Autodesk Inventor part; units mm, degrees
ref_plane "YZ Plane" through (0, 0, 0) normal (1, 0, 0) x (0, 1, 0)
ref_plane "XZ Plane" through (0, 0, 0) normal (0, 1, 0) x (-1, 0, 0)
ref_plane "XY Plane" through (0, 0, 0) normal (0, 0, 1) x (1, 0, 0)
sketch "Sketch1" plane through (0, 0, 0) normal (0, 1, 0) x (-1, 0, 0)
  circle A0 centre (0, 0) radius 25
  circle A1 centre (-200, 0) radius 25
  line L0 (0, 25) -> (-200, 25)
  line L1 (-200, 25) -> (-200, -25)
  line L2 (-200, -25) -> (0, -25)
  line L3 (0, -25) -> (0, 25)
  point P0 (-200, 0)
  point P1 (0, 0)
  point P2 (0, -25)
  dimension "d0" = 50
  dimension "d1" = 50
  dimension "d2" = 200
extrude "Extrusion1" add sketch "Sketch1" along normal mid plane 20
sketch "Sketch4" plane through (0, 0, 0) normal (0, 1, 0) x (-1, 0, 0)
  arc A0 (0, -25) -> (0, 25) centre (0, 0) ccw
  line L0 (0, -25) -> (-200, -25)
  arc A1 (-200, 25) -> (-200, -25) centre (-200, 0) ccw
  line L1 (-200, 25) -> (0, 25)
  line L2 (0, -25) -> (-200, -25)
  line L3 (-80, -25) -> (-80, 25)
  line L4 (-200, 25) -> (0, 25)
  dimension "d10" = 80
extrude "Extrusion3" add sketch "Sketch4" along normal mid plane 50 contours L0 L3 L1 A0
sketch "Sketch6" plane through (0, 0, 0) normal (0, 1, 0) x (-1, 0, 0)
  circle A0 centre (0, 0) radius 15
  arc A1 (-200, 25) -> (-200, -25) centre (-200, 0) ccw
  circle A2 centre (-200, 0) radius 15
  line L0 (0, -25) -> (-80, -25)
  line L1 (-65, -25) -> (-65, 25)
  arc A3 (0, -25) -> (0, 25) centre (0, 0) ccw
  line L2 (-80, 25) -> (0, 25)
  point P0 (-65, 0)
  point P1 (25, 0)
  dimension "d13" = 30
  dimension "d14" = 30
  dimension "d16" = 90
extrude "Extrusion4" cut sketch "Sketch6" along normal mid plane 20
properties part number "Manipulator Link"
Could you check a few things on this model? Use its own coordinates, in mm. A direction names the side the tool comes from. Give positions to 0.01 mm unless a question says otherwise; leave off trailing zeros. Loops run counter-clockwise (first coordinate to the right, second up) from the corner with the lowest first, then second, coordinate; pieces in that order, holes last. Notation, with made-up numbers: M 55,76 L 88,76 A23 cw 88,92 Z; hole C 67.5,-3 d11. An arc over 180 degrees is marked long. Answer as a JSON object with one key per item and string values.
Q1. If I drill on probe 1 along X at (y, z) = (3, 1); probe 2 along Z at (x, y) = (200, 1); probe 3 along Y at (x, z) = (9.5, -12.5), over which ranges is the centre line in solid material (lowest first)? Write a range as [from, to].
Values found:
{"probe 1": "x = [-14.97, 14.97], [65, 185.03], [214.97, 224.98]", "probe 2": "z = [-25, -15], [15, 25]", "probe 3": "y = [-25, -10], [10, 25]"}
Q2. Suppose I cut it at D-D, the plane x = 165.5. List the corners of the cut face in (y, z) for me.
Values found:
{"outline": "M -10,-25 L 10,-25 L 10,25 L -10,25 Z"}
Q3. For P1, Ø3, axis at y = -12.5, z = 0.5, coming from the +X side; P2, Ø8, axis at x = 150, z = 2, coming from the +Y side; P3, Ø6, axis at y = 1.5, z = 12, coming from the -X side, each with a flat end and sliding along its axis, tell me the tip position at first contact or that it passes through.
Values found:
{"P1": "stops at x = 80", "P2": "stops at y = 10", "P3": "stops at x = -12"}
Q4. If we mould it in two halves opening along Y, with no side actions, what happens to faces 1 (the cylindrical face through (224.994, -0.14, -0.55)), 2 (the flat face through (154, 10, 0)), 3 (the flat face through (31, 10, 0))? For each: pulls with the +Y half, pulls with the -Y half, needs draft (parallel to the pull), parting line crosses it, or undercut.
Values found:
{"face 1": "needs draft", "face 2": "pulls with the +Y half", "face 3": "undercut"}
Q5. Suppose I cut it at A-A, the plane z = 0. List the corners of the cut face in (x, y) for me.
Values found:
{"outline": "M -25,-25 L 80,-25 L 80,-10 L 185,-10 L 185,10 L 80,10 L 80,25 L -25,25 L -25,10 L -15,10 L -15,-10 L -25,-10 Z; M 215,-10 L 225,-10 L 225,10 L 215,10 Z; hole M 15,-10 L 65,-10 L 65,10 L 15,10 Z"}
Q6. For faces 4 (the cylindrical face through (14.985, -0.14, -0.66)), 5 (the flat face through (80, 17, 0)), 6 (the flat face through (65, 0, 0)), 7 (the flat face through (80, -18, 0)), which set-ups out of +Z, -Z, +X, -X, +Y, -Y let a thin tool reach every point of the face, with its end or its side?
Values found:
{"face 4": "none", "face 5": "+Z, -Z, +X, +Y", "face 6": "+Z, -Z", "face 7": "+Z, -Z, +X, -Y"}
Q7. Suppose I cut it at C-C, the plane z = 10. List the corners of the cut face in (x, y) for me.
Values found:
{"outline": "M -22.91,-25 L 80,-25 L 80,-10 L 188.82,-10 L 188.82,10 L 80,10 L 80,25 L -22.91,25 L -22.91,10 L -11.18,10 L -11.18,-10 L -22.91,-10 Z; M 211.18,-10 L 222.91,-10 L 222.91,10 L 211.18,10 Z; hole M 11.18,-10 L 65,-10 L 65,10 L 11.18,10 Z"}
Q8. Suppose I cut it at B-B, the plane y = -4. List the corners of the cut face in (x, z) for me.
Values found:
{"outline": "C 0,0 d30; M 65,-25 L 200,-25 A25 ccw 200,25 L 65,25 Z; hole C 200,0 d30"}
